The drawing under review shows one solid part. Ordinate dimensions are in mm from its lowest x, y, z. A direction names the side the tool comes from. Give positions to 0.01 mm unless a question says otherwise; leave off trailing zeros. Loops run counter-clockwise (first coordinate to the right, second up) from the corner with the lowest first, then second, coordinate; pieces in that order, holes last.
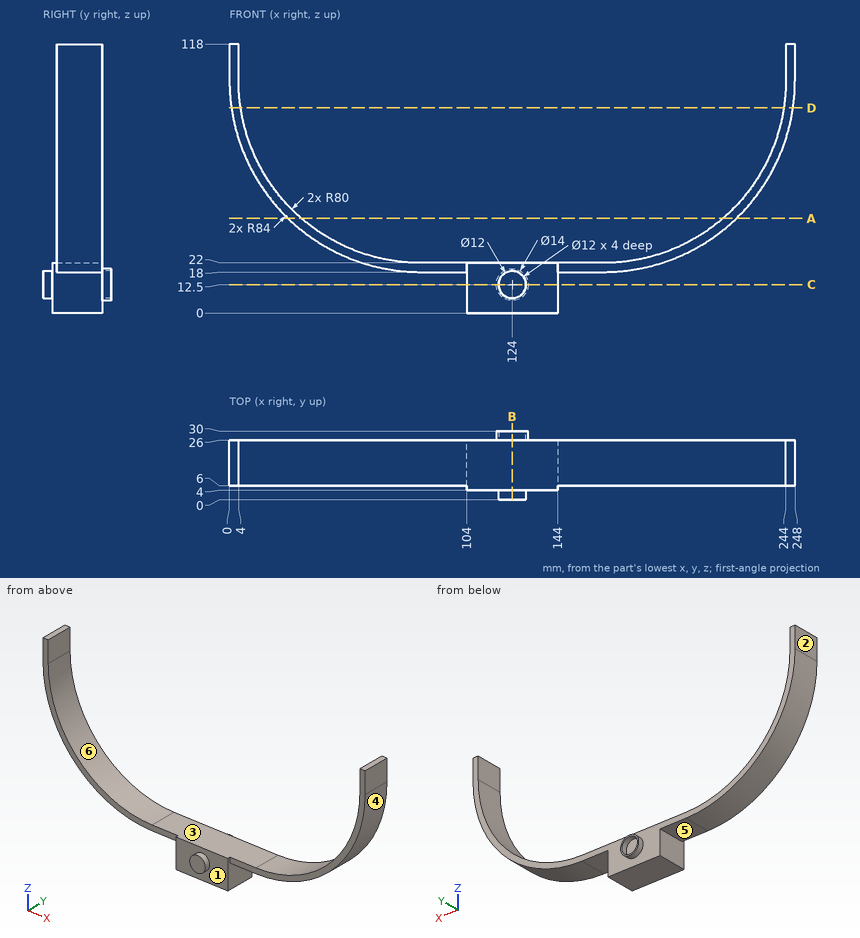
Item 1: Take a section at D-D on z = 90. Give the boundary of the cut face in (x, y), and give its area (3 significant figures).
Answer:
outline: (0.86, 6) - (4.91, 6) - (4.91, 26) - (0.86, 26) - close; (243.09, 6) - (247.14, 6) - (247.14, 26) - (243.09, 26) - close
area: 162 mm2
Item 2: Clearance check with flat-ended pins moving along their axes: pin 1 Ø5 at (x, y) = (212.5, 5.5) entering from -Z; pin 2 Ø12 at (x, y) = (143.5, 9.5) entering from +Z; pin 3 Ø8 at (x, y) = (84, 18.5) entering from +Z. State where each tip first meets the part, or that it passes through.
Answer:
pin 1: stops at z = 31.75
pin 2: stops at z = 22
pin 3: stops at z = 22.1
Item 3: For L1, parallel to Z at x = 124, y = 26.95; L2, parallel to X at y = 10.25, z = 111; L3, parallel to X at y = 27.2, z = 12.5, list the stretches that pass through material, from the lowest coordinate up.
Answer:
L1: z = 5.5 to 6.5, 18.5 to 19.5
L2: x = 0 to 4, 244 to 248
L3: x = 117 to 118, 130 to 131
Item 4: Take a section at A-A on z = 41.5. Give the boundary of the cut face in (x, y), and give its area (3 significant figures).
Answer:
outline: (25.73, 6) - (31.66, 6) - (31.66, 26) - (25.73, 26) - close; (216.34, 6) - (222.27, 6) - (222.27, 26) - (216.34, 26) - close
area: 237 mm2
Item 5: Take a section at C-C on z = 12.5. Give the boundary of the cut face in (x, y), and give its area (3 significant figures).
Answer:
outline: (104, 4) - (118, 4) - (118, 0) - (130, 0) - (130, 4) - (144, 4) - (144, 26) - (131, 26) - (131, 30) - (130, 30) - (130, 26) - (118, 26) - (118, 30) - (117, 30) - (117, 26) - (104, 26) - close
area: 936 mm2
Item 6: Tool access review of the marked faces 4, 5 and 6: name each direction out of +Z, -Z, +X, -X, +Y, -Y from which nothing blocks a thin tool from reaching the whole face with its end or side.
Answer:
face 4: -Z, +X, +Y, -Y
face 5: -Z, -X, +Y, -Y
face 6: +Z, +Y, -Y
Item 7: Take a section at B-B on x = 124. Give the boundary of the cut face in (y, z).
Answer:
outline: (0, 6.5) - (4, 6.5) - (4, 0) - (26, 0) - (26, 5.5) - (30, 5.5) - (30, 6.5) - (26, 6.5) - (26, 18.5) - (30, 18.5) - (30, 19.5) - (26, 19.5) - (26, 22) - (4, 22) - (4, 18.5) - (0, 18.5) - close
Item 8: The part is to be moulded in two halves that separate along X. For the marked faces 1, 2 and 3, say which applies: released by +X, released by -X, zero draft, split by the parting line, or undercut.
Answer:
face 1: zero draft
face 2: released by -X
face 3: undercut
